Build history of the part. All positions in model axes, mm. Face numbers are marked on the shaded views. A direction names the side the tool comes from. Give positions to 0.01 mm unless a question says otherwise; leave off trailing zeros. Loops run counter-clockwise (first coordinate to the right, second up) from the corner with the lowest first, then second, coordinate; pieces in that order, holes last. Notation, with made-up numbers: (-5, 0) -> (45, 0) arc R19 cw to (45, 13) -> close; hole circle Ø10 at (5, -16). An arc over 180 degrees is marked (long way). Answer as a JSON object with one key per item and string values. Group by question number.
Q1. Band-saw the part on B-B, the plane x = 10. Write the cut outline in (y, z).
Q2. Wall check: probe 1 along Y at (x, z) = (13, -34); probe 2 along Y at (x, z) = (14, -17); probe 3 along Y at (x, z) = (4.5, -17.5). Give the ranges that are in metal, low to high. Write a range as from..to.
Q3. Band-saw the part on A-A, the plane z = -30.5. Write the cut outline in (x, y), plus the area to 3 significant figures.
Q4. Two-plate mould, pull along Y, no slides. Class the marked faces 4, 5 and 6: pulls with the +Y half, pulls with the -Y half, needs draft (parallel to the pull), parting line crosses it, or undercut.
Q5. Band-saw the part on D-D, the plane y = 11. Write the cut outline in (x, z).
Q6. Band-saw the part on C-C, the plane z = -51. Write the cut outline in (x, y), plus the area to 3 significant figures.
Q7. Drop flat-ended pins along their axis: pin 1 (5 mm diameter, centred on x = 5.5, y = 112.5, fed in from -Z); pin 2 (2 mm diameter, centred on x = 11.5, y = 98.5, fed in from +Z); pin 3 (2 mm diameter, centred on x = 17.5, y = 107, fed in from +Z); pin 4 (8 mm diameter, centred on x = 14.5, y = 105, fed in from +Z). Give the stop position or say it passes through.
Q8. Tool access for the marked faces 1, 2 and 3: list every direction of +Z, -Z, +X, -X, +Y, -Y with a clear straight run to the whole face (end or side of a thin tool).
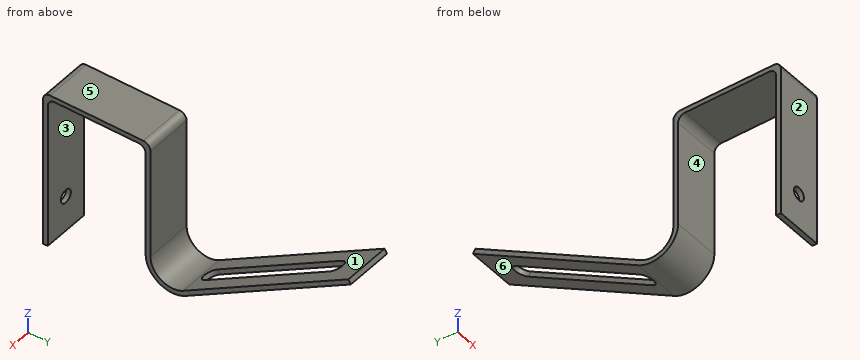
from build123d import *

# Parameters (mm, degrees)
RESSALTO_EXTRUS_O4_DEPTH = 20
FILETE1_R                = 3
ESBO_O5_R                = 2.75
CORTE_EXTRUS_O1_DEPTH    = 2
CORTE_EXTRUS_O2_DEPTH    = 2


with BuildPart() as part:
    # Esboço4 → Ressalto-extrusão4 (new body)
    with BuildSketch(Plane(origin=(0, 0, 0), x_dir=(0, 0, -1), z_dir=(1, 0, 0))):
        with BuildLine():
            Line((0, 0), (66, 0))
            Line((66, 0), (66, 2))
            Line((66, 2), (2, 2))
            Line((2, 2), (2, 43))
            Line((2, 43), (49, 43))
            ThreePointArc((49, 43), (58.614151216, 48.550732793), (58.614151216, 59.652198378))
            Line((58.614151216, 59.652198378), (18.614151216, 128.93423068))
            Line((18.614151216, 128.93423068), (16.882100408, 127.93423068))
            Line((16.882100408, 127.93423068), (56.882100408, 58.652198378))
            ThreePointArc((56.882100408, 58.652198378), (56.882100408, 49.550732793), (49, 45))
            Line((49, 45), (0, 45))
            Line((0, 45), (0, 0))
        make_face()
    extrude(amount=RESSALTO_EXTRUS_O4_DEPTH)

    # Filete1
    filete1_edges = [part.edges().sort_by_distance(p)[0] for p in [
        (10, 45, 0),
        (10, 43, -2),
        (10, 2, -2),
        (10, 0, 0),
    ]]
    fillet(filete1_edges, radius=FILETE1_R)

    # Esboço5 → Corte-extrusão1 (cut)
    with BuildSketch(Plane.XZ):
        with Locations(Location((10, -51, 0), (0, 0, 270))):
            Circle(ESBO_O5_R)
    extrude(amount=-CORTE_EXTRUS_O1_DEPTH, mode=Mode.SUBTRACT)

    # Esboço6 → Corte-extrusão2 (cut)
    with BuildSketch(Plane(origin=(0, 40.293721582, -69.790773005), x_dir=(-1, 0, 0), z_dir=(0, 0.4999999999999983, -0.8660254037844398))):
        with BuildLine():
            Line((-13.5, 87.353243579), (-13.5, 27.353243579))
            ThreePointArc((-13.5, 27.353243579), (-10, 23.853243579), (-6.5, 27.353243579))
            Line((-6.5, 27.353243579), (-6.5, 87.353243579))
            ThreePointArc((-6.5, 87.353243579), (-10, 90.853243579), (-13.5, 87.353243579))
        make_face()
    extrude(amount=-CORTE_EXTRUS_O2_DEPTH, mode=Mode.SUBTRACT)


solid = part.part
Worked answers:
{
 "1": {"outline": "(0, -66) -> (2, -66) -> (2, -53.75) -> (0, -53.75) -> close; (0, -48.25) -> (2, -48.25) -> (2, -5) arc R3 cw to (5, -2) -> (40, -2) arc R3 cw to (43, -5) -> (43, -49) arc R11.1 ccw to (59.65, -58.61) -> (60.95, -57.86) -> (59.95, -56.13) -> (58.65, -56.88) arc R9.1 cw to (45, -49) -> (45, -3) arc R3 ccw to (42, 0) -> (3, 0) arc R3 ccw to (0, -3) -> close; (117.97, -22.63) -> (118.97, -24.36) -> (128.93, -18.61) -> (127.93, -16.88) -> close"},
 "2": {"probe 1": "0..2, 43..45", "probe 2": "0..2, 43..45, 127.73..128", "probe 3": "0..2, 43..45, 126.86..128.29"},
 "3": {"outline": "(0, 0) -> (20, 0) -> (20, 2) -> (0, 2) -> close; (0, 43) -> (20, 43) -> (20, 45) -> (0, 45) -> close; (0, 104.35) -> (6.5, 104.35) -> (6.5, 108.35) -> (0, 108.35) -> close; (13.5, 104.35) -> (20, 104.35) -> (20, 108.35) -> (13.5, 108.35) -> close", "area": "132 mm2"},
 "4": {"face 4": "undercut", "face 5": "needs draft", "face 6": "pulls with the +Y half"},
 "5": {"outline": "(0, -2) -> (20, -2) -> (20, 0) -> (0, 0) -> close"},
 "6": {"outline": "(0, 0) -> (7.25, 0) -> (7.25, 2) -> (0, 2) -> close; (0, 43.18) -> (20, 43.18) -> (20, 45.22) -> (0, 45.22) -> close; (0, 68.84) -> (6.5, 68.84) -> (6.5, 72.84) -> (0, 72.84) -> close; (12.75, 0) -> (20, 0) -> (20, 2) -> (12.75, 2) -> close; (13.5, 68.84) -> (20, 68.84) -> (20, 72.84) -> (13.5, 72.84) -> close", "area": "122 mm2"},
 "7": {"pin 1": "z = -29.55", "pin 2": "through", "pin 3": "z = -28.39", "pin 4": "z = -27.81"},
 "8": {"face 1": "+Z, +X, -X", "face 2": "+Z, -Z, +X, -X, -Y", "face 3": "-Z, +X, -X"}
}
